Autodesk Inventor part; units mm, degrees
ref_plane "YZ Plane" through (0, 0, 0) normal (1, 0, 0) x (0, 1, 0)
ref_plane "XZ Plane" through (0, 0, 0) normal (0, 1, 0) x (-1, 0, 0)
ref_plane "XY Plane" through (0, 0, 0) normal (0, 0, 1) x (1, 0, 0)
sketch "Sketch1" plane through (0, 0, 0) normal (0, 0, 1) x (1, 0, 0)
  line L0 (-362.4815, -406.4) -> (399.5185, -406.4)
  line L1 (399.5185, -406.4) -> (399.5185, 406.4)
  line L2 (399.5185, 406.4) -> (-362.4815, 406.4)
  line L3 (-362.4815, 406.4) -> (-362.4815, -406.4)
  point P0 (0, 0)
extrude "Extrusion1" add sketch "Sketch1" along normal blind 150.114
sketch "Sketch3" plane through (0, 0, 150.114) normal (0, 0, 1) x (1, 0, 0)
  line L0 (-356.7823, 401.8579) -> (395.0577, 401.8579)
  line L1 (395.0577, 401.8579) -> (395.0577, -400.7821)
  line L2 (395.0577, -400.7821) -> (-356.7823, -400.7821)
  line L3 (-356.7823, -400.7821) -> (-356.7823, 401.8579)
  point P0 (0, 0)
  dimension "d10" = 751.84
  dimension "d11" = 802.64
extrude "Extrusion2" cut sketch "Sketch3" against normal blind 139.7
sketch "Sketch4" plane through (0, 0, 0) normal (0, 0, -1) x (-1, 0, 0)
  line L0 (-345.9489, 321.1782) -> (-25.9089, 321.1782)
  line L1 (-25.9089, 321.1782) -> (-25.9089, -318.9018)
  line L2 (-25.9089, -318.9018) -> (-345.9489, -318.9018)
  line L3 (-345.9489, -318.9018) -> (-345.9489, 321.1782)
  line L4 (140.3393, 137.685) -> (240.6693, 137.685)
  line L5 (240.6693, 137.685) -> (240.6693, 90.4401)
  line L6 (240.6693, 90.4401) -> (140.3393, 90.4401)
  line L7 (140.3393, 90.4401) -> (140.3393, 137.685)
  line L8 (139.7596, 266.0514) -> (240.0896, 266.0514)
  line L9 (240.0896, 266.0514) -> (240.0896, 218.8065)
  line L10 (240.0896, 218.8065) -> (139.7596, 218.8065)
  line L11 (139.7596, 218.8065) -> (139.7596, 266.0514)
  point P0 (0, 0)
  dimension "d17" = 100.33
  dimension "d18" = 47.2449
  dimension "d19" = 100.33
  dimension "d20" = 47.2449
extrude "Extrusion3" cut sketch "Sketch4" against normal blind 279.4
properties part number "tetris body"
Check sheet for the modelled part. Datum: model origin and axes. Units: mm. A direction names the side the tool comes from. Round coordinates to 2 decimals unless told otherwise and drop trailing zeros. Loops run counter-clockwise (first coordinate to the right, second up) from the corner with the lowest first, then second, coordinate; pieces in that order, holes last.
1. Gauge pin test, flat end, axial feed: pin 1 Ø1 at (x, y) = (-124.5, 146) entering from +Z. Record the tip position at first contact, or that the pin passes through.
2. Sectioned sample at C-C on z = 80.5. Record the boundary of the cut face in (x, y).
3. Sectioned sample at A-A on x = 140.5. Record the boundary of the cut face in (y, z).
4. Scan lines: probe 1 along X at (y, z) = (-102.5, 46.5); probe 2 along Y at (x, z) = (304.5, 36); probe 3 along Z at (x, y) = (367.5, 110). Record each from-to range of solid material in increasing order.
5. Sectioned sample at B-B on y = 185.5. Record the boundary of the cut face in (x, z).
6. Set-up check for faces 5 (the flat face through (-71, 6, 0)), 6 (the flat face through (24, -400.782, 81)): record each of +Z, -Z, +X, -X, +Y, -Y from which the full face is reachable in a straight line by a thin tool's end or side.
7. Mould release check, pull along X, two halves, no side actions. Record for faces 1 (the flat face through (24, 406.4, 74)), 2 (the flat face through (-362.482, 6, 74)), 3 (the flat face through (395.058, 6, 81)), 4 (the flat face through (399.518, -6, 74)): released by +X, released by -X, zero draft, split by the parting line, or undercut.
8. Sectioned sample at D-D on y = 102. Record the boundary of the cut face in (x, z), and give its area (3 significant figures).
Recorded:
1. pin 1: stops at z = 10.41
2. outline: (-362.48, -406.4) - (399.52, -406.4) - (399.52, 406.4) - (-362.48, 406.4) - close; hole (-356.78, -400.78) - (395.06, -400.78) - (395.06, 401.86) - (-356.78, 401.86) - close
3. outline: (-406.4, 0) - (-318.9, 0) - (-318.9, 10.41) - (-400.78, 10.41) - (-400.78, 150.11) - (-406.4, 150.11) - close; (321.18, 0) - (406.4, 0) - (406.4, 150.11) - (401.86, 150.11) - (401.86, 10.41) - (321.18, 10.41) - close
4. probe 1: x = -362.48 to -356.78, 395.06 to 399.52
4. probe 2: y = -406.4 to -400.78, 401.86 to 406.4
4. probe 3: z = 0 to 10.41
5. outline: (-362.48, 0) - (25.91, 0) - (25.91, 10.41) - (-356.78, 10.41) - (-356.78, 150.11) - (-362.48, 150.11) - close; (345.95, 0) - (399.52, 0) - (399.52, 150.11) - (395.06, 150.11) - (395.06, 10.41) - (345.95, 10.41) - close
6. face 5: -Z, +X, -X, +Y, -Y
6. face 6: +Z
7. face 1: zero draft
7. face 2: released by -X
7. face 3: undercut
7. face 4: released by +X
8. outline: (-362.48, 0) - (-240.67, 0) - (-240.67, 10.41) - (-356.78, 10.41) - (-356.78, 150.11) - (-362.48, 150.11) - close; (-140.34, 0) - (25.91, 0) - (25.91, 10.41) - (-140.34, 10.41) - close; (345.95, 0) - (399.52, 0) - (399.52, 150.11) - (395.06, 150.11) - (395.06, 10.41) - (345.95, 10.41) - close
8. area: 4,980 mm2
